Autodesk Inventor part; units mm, degrees
ref_plane "YZ Plane" through (0, 0, 0) normal (1, 0, 0) x (0, 1, 0)
ref_plane "XZ Plane" through (0, 0, 0) normal (0, 1, 0) x (-1, 0, 0)
ref_plane "XY Plane" through (0, 0, 0) normal (0, 0, 1) x (1, 0, 0)
sketch "Szkic1" plane through (0, 0, 0) normal (1, 0, 0) x (0, 1, 0)
  line L0 (0, 0) -> (10, 0)
  line L1 (10, 0) -> (10, -3.6)
  line L2 (10, -3.6) -> (15, -3.6)
  line L3 (15, -3.6) -> (15, -7.4)
  line L4 (15, -7.4) -> (13, -7.4)
  line L5 (13, -7.4) -> (13, -6)
  line L6 (13, -6) -> (0, -6)
  line L7 (0, -6) -> (0, 0)
  dimension "d1" = 2.4
  dimension "d2" = 3.8
  dimension "d3" = 2
  dimension "d4" = 3.6
  dimension "d5" = 5
  dimension "d6" = 15
extrude "Wyciągnięcie proste1" add sketch "Szkic1" along normal blind 30
fillet "Zaokrąglenie1" radius 3 1 edges at (15, 0, 0)
fillet "Zaokrąglenie2" radius 1 5 edges at (15, 15, -3.6) (15, 10, -3.6) (15, 15, -7.4) (15, 13, -7.4) (15, 13, -6)
sketch "Szkic4" plane through (0, 10, 0) normal (0, 0, 1) x (1, 0, 0)
  line L0 (30, -7) -> (0, -7)
  line L1 (30, 0) -> (30, -7)
  line L2 (0, 0) -> (30, 0) construction
  line L3 (0, 0) -> (0, -7)
  circle A0 centre (25, -5) radius 0.75
  circle A1 centre (15, -5) radius 0.75
  circle A2 centre (5, -5) radius 0.75
  dimension "d27" = 1.5
  dimension "d28" = 2
  dimension "d32" = 10
  dimension "d38" = 30
  dimension "d39" = 15
extrude "Wyciągnięcie proste5" cut sketch "Szkic4" against normal through all
equation "\"d39\" = 0.5 * d38"
properties part number "paliczek_v2" material "PLA"
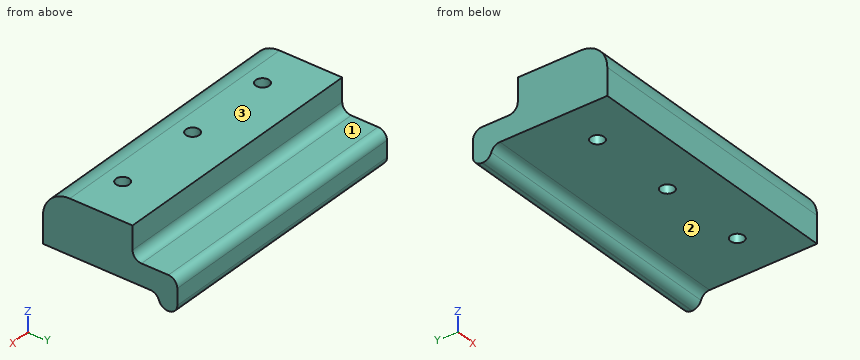
Design review of the part built by this model. Coordinates are the model's own, in mm. Face numbers are marked on the shaded views. A direction names the side the tool comes from. Give positions to 0.01 mm unless a question says otherwise; leave off trailing zeros. Order: outer loops, then holes, each group sorted by start corner. A loop starts at its lowest first (then second) coordinate and runs counter-clockwise, first axis right, second up.
1. Add section C-C, the plane z = -1.25. State the section outline as (x, y) points.
Solution:
outline: (0, 0.56) - (30, 0.56) - (30, 10) - (0, 10) - close; hole circle Ø1.5 at (5, 5); hole circle Ø1.5 at (15, 5); hole circle Ø1.5 at (25, 5)
2. Add section D-D, the plane y = 10.5. State the section outline as (x, z) points.
Solution:
outline: (0, -6) - (30, -6) - (30, -3.47) - (0, -3.47) - close
3. Add section B-B, the plane z = -4. State the section outline as (x, y) points.
Solution:
outline: (0, 0) - (30, 0) - (30, 14.8) - (0, 14.8) - close; hole circle Ø1.5 at (5, 5); hole circle Ø1.5 at (15, 5); hole circle Ø1.5 at (25, 5)
4. To check wall thickness, follow L1, parallel to X at y = 4.5, z = -5.75; L2, parallel to Y at x = 25, z = -4.75; L3, parallel to Z at x = 26, y = 4.75. State the ranges of each line that lie inside material, in increasing order.
Solution:
L1: x = 0 to 4.44, 5.56 to 14.44, 15.56 to 24.44, 25.56 to 30
L2: y = 0 to 4.25, 5.75 to 15
L3: z = -6 to 0
5. For pin 1 Ø2 at (x, z) = (8, -1.5) entering from +Y; pin 2 Ø0.9 at (x, y) = (17, 12) entering from +Z; pin 3 Ø2.5 at (x, y) = (25, 5) entering from +Z, all flat-tipped, find the tip position at first contact; note any pin that passes through.
Solution:
pin 1: stops at y = 10
pin 2: stops at z = -3.6
pin 3: stops at z = 0
6. Add section A-A, the plane y = 5. State the section outline as (x, z) points.
Solution:
outline: (0, -6) - (4.25, -6) - (4.25, 0) - (0, 0) - close; (5.75, -6) - (14.25, -6) - (14.25, 0) - (5.75, 0) - close; (15.75, -6) - (24.25, -6) - (24.25, 0) - (15.75, 0) - close; (25.75, -6) - (30, -6) - (30, 0) - (25.75, 0) - close
7. Tool access review of the marked faces 1, 2 and 3: name each direction out of +Z, -Z, +X, -X, +Y, -Y from which nothing blocks a thin tool from reaching the whole face with its end or side.
Solution:
face 1: +Z, +X, -X, +Y
face 2: -Z, +X, -X, -Y
face 3: +Z, +X, -X, +Y, -Y
